Design review of the part built by this model. Coordinates are the model's own, in mm. Give positions to 0.01 mm unless a question says otherwise; leave off trailing zeros. Write each loop counter-clockwise with the first axis right and the second up, starting at its lowest first coordinate (ties: lowest second). Pieces come first, ordered by that corner, then holes. Notation, with made-up numbers: M 2,9.25 L 14,9.25 A12 cw 14,26.25 Z; hole C 9,-21.5 d7. An arc over 180 degrees is marked long. One line per item, written item: value. Start each with the question number.
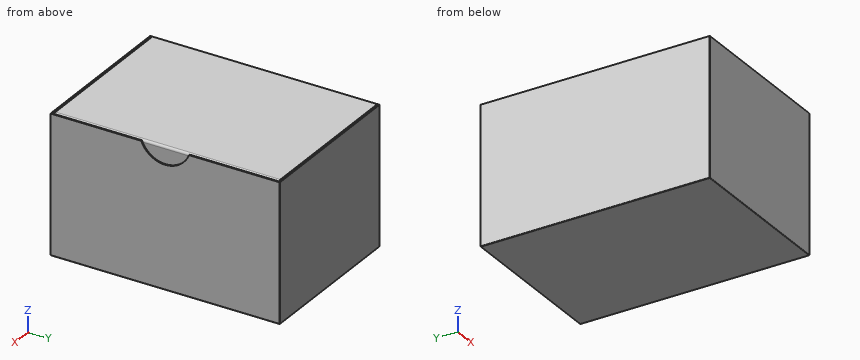
```python
from build123d import *

# Parameters (mm, degrees)
F0_W     = 70
F0_H     = 100
F1_DEPTH = 60
F2_R     = 0.2
F3_T     = -0.5
F4_W     = 68.5
F4_H     = 98
F5_DEPTH = 0.5
F6_DEPTH = 10
F7_R     = 1
F9_DEPTH = 0.5


with BuildPart() as f1:
    # F0 (on Top) → F1 (new body)
    with BuildSketch(Plane.XY):
        Rectangle(F0_W, F0_H)
    extrude(amount=F1_DEPTH)

    # F2
    f2_edges = [f1.edges().sort_by_distance(p)[0] for p in [
        (35, -50, 30),
        (35, 0, 0),
        (0, 50, 0),
        (-35, 0, 0),
        (0, -50, 0),
        (35, 50, 30),
        (-35, 50, 30),
        (-35, -50, 30),
    ]]
    fillet(f2_edges, radius=F2_R)

    # F3
    f3_openings = [f1.faces().sort_by_distance(p)[0] for p in [
        (0, 0, 60),
    ]]
    offset(amount=F3_T, openings=f3_openings)

    # F4 (on face) → F5 (join)
    with BuildSketch(Plane.XY.offset(60)):
        with Locations((-0.25, 0)):
            Rectangle(F4_W, F4_H)
    extrude(amount=-F5_DEPTH)

    # F4 (on face) → F6 (join)
    with BuildSketch(Plane.XY.offset(60)):
        with Locations((-0.25, 0)):
            Rectangle(F4_W, F4_H)
    extrude(amount=-F6_DEPTH)

    # F7
    f7_edges = [f1.edges().sort_by_distance(p)[0] for p in [
        (34, 0, 60),
    ]]
    fillet(f7_edges, radius=F7_R)

    # F8 (on face) → F9 (cut)
    with BuildSketch(Plane.YZ.offset(35)):
        with BuildLine():
            Line((10.426263, 60), (-10.426263, 60))
            ThreePointArc((-10.426263, 60), (0, 52.880268), (10.426263, 60))
        make_face()
    extrude(amount=-F9_DEPTH, mode=Mode.SUBTRACT)


solid = f1.part
```
Q1. Take a section at A-A, the plane x = 14.5. Give the boundary of the cut face in (y, z).
Q2. Wall thickness on line 1 (Y direction, x = -7, z = 55); line 2 (X direction, y = -21, z = 9); line 3 (Y direction, x = -1, z = 48): over which ranges is each line inside the solid? List them lowest first. Write a range as from..to.
Q3. Take a section at D-D, the plane z = 55.5. Give the boundary of the cut face in (x, y).
Q4. Take a section at B-B, the plane z = 22. Give the boundary of the cut face in (x, y), then the cut area to 3 significant figures.
Q5. Take a section at C-C, the plane y = 9. Give the boundary of the cut face in (x, z).
Results list:
1. outline: M -50,0.2 A0.2 ccw -49.8,0 L 49.8,0 A0.2 ccw 50,0.2 L 50,60 L 49.5,60 L 49.5,0.5 L -49.5,0.5 L -49.5,60 L -50,60 Z; M -49,50 L 49,50 L 49,60 L -49,60 Z
2. line 1: y = -50..-49.5, -49..49, 49.5..50
2. line 2: x = -35..-34.5, 34.5..35
2. line 3: y = -50..-49.5, 49.5..50
3. outline: M -35,-49.8 A0.2 ccw -34.8,-50 L 34.8,-50 A0.2 ccw 35,-49.8 L 35,-7.2 L 34.5,-7.2 L 34.5,-49.5 L -34.5,-49.5 L -34.5,-49 L 34,-49 L 34,49 L -34.5,49 L -34.5,49.5 L 34.5,49.5 L 34.5,7.2 L 35,7.2 L 35,49.8 A0.2 ccw 34.8,50 L -34.8,50 A0.2 ccw -35,49.8 Z
4. outline: M -35,-49.8 A0.2 ccw -34.8,-50 L 34.8,-50 A0.2 ccw 35,-49.8 L 35,49.8 A0.2 ccw 34.8,50 L -34.8,50 A0.2 ccw -35,49.8 Z; hole M -34.5,-49.5 L 34.5,-49.5 L 34.5,49.5 L -34.5,49.5 Z
4. area: 169 mm^2
5. outline: M -35,0.2 A0.2 ccw -34.8,0 L 34.8,0 A0.2 ccw 35,0.2 L 35,57.42 L 34.5,57.42 L 34.5,0.5 L -34.5,0.5 L -34.5,50 L 34,50 L 34,59 A1 ccw 33,60 L -35,60 Z
